from build123d import *

# Parameters (mm, degrees)
CROQUIS2_W                 = 25
CROQUIS2_H                 = 50
SALIENTE_EXTRUIR1_DEPTH    = 800
SALIENTE_EXTRUIR1_2_DEPTH  = 800
SALIENTE_EXTRUIR1_3_DEPTH  = 800
SALIENTE_EXTRUIR1_4_DEPTH  = 800
CROQUIS3_W                 = 25
CROQUIS3_H                 = 50
SALIENTE_EXTRUIR2_DEPTH    = 230
CROQUIS4_W                 = 25
CROQUIS4_H                 = 50
SALIENTE_EXTRUIR3_DEPTH    = 65
CROQUIS5_W                 = 25
CROQUIS5_H                 = 50
SALIENTE_EXTRUIR4_DEPTH    = 65
CROQUIS6_W                 = 25
CROQUIS6_H                 = 50
SALIENTE_EXTRUIR5_DEPTH    = 800
CROQUIS7_W                 = 25
CROQUIS7_H                 = 50
SALIENTE_EXTRUIR6_DEPTH    = 270
CROQUIS8_W                 = 25
CROQUIS8_H                 = 50
SALIENTE_EXTRUIR7_DEPTH    = 180
CROQUIS9_W                 = 625
CROQUIS9_H                 = 180
CROQUIS9_W_2               = 125
CORTAR_EXTRUIR1_DEPTH      = 201
CORTAR_EXTRUIR1_DEPTH_BACK = 201


with BuildPart() as part:
    # Croquis2 → Saliente-Extruir1 (new body)
    with BuildSketch(Plane.XY):
        with Locations((-187.5, 25)):
            Rectangle(CROQUIS2_W, CROQUIS2_H)
    extrude(amount=SALIENTE_EXTRUIR1_DEPTH)



with BuildPart() as body_2:
    # Croquis2 → Saliente-Extruir1 2 (new body)
    with BuildSketch(Plane.XY):
        with Locations((187.5, 25)):
            Rectangle(CROQUIS2_W, CROQUIS2_H)
    extrude(amount=SALIENTE_EXTRUIR1_2_DEPTH)


with BuildPart() as body_3:
    # Croquis2 → Saliente-Extruir1 3 (new body)
    with BuildSketch(Plane.XY):
        with Locations((-122.5, 25)):
            Rectangle(CROQUIS2_W, CROQUIS2_H)
    extrude(amount=SALIENTE_EXTRUIR1_3_DEPTH)



with BuildPart() as body_4:
    # Croquis2 → Saliente-Extruir1 4 (new body)
    with BuildSketch(Plane.XY):
        with Locations((122.5, 25)):
            Rectangle(CROQUIS2_W, CROQUIS2_H)
    extrude(amount=SALIENTE_EXTRUIR1_4_DEPTH)


with BuildPart() as body_3_1:
    add(body_3.part)

    add(body_4.part)  # Saliente-Extruir2 merges body 4
    # Croquis3 → Saliente-Extruir2 (add)
    with BuildSketch(Plane.XZ):
        with Locations((-122.5, 775)):
            Rectangle(CROQUIS3_W, CROQUIS3_H)
        with Locations((122.5, 775)):
            Rectangle(CROQUIS3_W, CROQUIS3_H)
        with Locations((-122.5, 25)):
            Rectangle(CROQUIS3_W, CROQUIS3_H)
        with Locations((122.5, 25)):
            Rectangle(CROQUIS3_W, CROQUIS3_H)
    extrude(amount=-SALIENTE_EXTRUIR2_DEPTH)


with BuildPart() as part_1:
    add(part.part)

    add(body_3_1.part)  # Saliente-Extruir3 merges body 3
    # Croquis4 → Saliente-Extruir3 (add)
    with BuildSketch(Plane.ZY.offset(200)):
        with Locations((12.5, 25)):
            Rectangle(CROQUIS4_W, CROQUIS4_H)
        with Locations((787.5, 25)):
            Rectangle(CROQUIS4_W, CROQUIS4_H)
    extrude(amount=-SALIENTE_EXTRUIR3_DEPTH)


    add(body_2.part)  # Saliente-Extruir4 merges body 2
    # Croquis5 → Saliente-Extruir4 (add)
    with BuildSketch(Plane(origin=(200, 0, 0), x_dir=(0, 0, -1), z_dir=(1, 0, 0))):
        with Locations((-787.5, 25)):
            Rectangle(CROQUIS5_W, CROQUIS5_H)
        with Locations((-12.5, 25)):
            Rectangle(CROQUIS5_W, CROQUIS5_H)
    extrude(amount=-SALIENTE_EXTRUIR4_DEPTH)

    # Croquis6 → Saliente-Extruir5 (add)
    with BuildSketch(Plane.XY.offset(800)):
        with Locations((-122.5, 205)):
            Rectangle(CROQUIS6_W, CROQUIS6_H)
        with Locations((122.5, 205)):
            Rectangle(CROQUIS6_W, CROQUIS6_H)
    extrude(amount=-SALIENTE_EXTRUIR5_DEPTH)

    # Croquis7 → Saliente-Extruir6 (add)
    with BuildSketch(Plane(origin=(135, 0, 0), x_dir=(0, 0, -1), z_dir=(1, 0, 0))):
        with Locations((-637.5, 205)):
            Rectangle(CROQUIS7_W, CROQUIS7_H)
    extrude(amount=-SALIENTE_EXTRUIR6_DEPTH)

    # Croquis8 → Saliente-Extruir7 (add)
    with BuildSketch(Plane(origin=(0, 230, 0), x_dir=(1, 0, 0), z_dir=(0, 1, 0))):
        with Locations((-122.5, -650)):
            Rectangle(CROQUIS8_W, CROQUIS8_H)
        with Locations((122.5, -650)):
            Rectangle(CROQUIS8_W, CROQUIS8_H)
    extrude(amount=-SALIENTE_EXTRUIR7_DEPTH)

    # Croquis9 → Cortar-Extruir1 (cut, two sides)
    with BuildSketch(Plane(origin=(0, 0, 0), x_dir=(0, 0, -1), z_dir=(1, 0, 0))) as cortar_extruir1_sk:
        with Locations((-312.5, 140)):
            Rectangle(CROQUIS9_W, CROQUIS9_H)
        with Locations((-737.5, 140)):
            Rectangle(CROQUIS9_W_2, CROQUIS9_H)
    extrude(amount=CORTAR_EXTRUIR1_DEPTH, mode=Mode.SUBTRACT)
    extrude(cortar_extruir1_sk.sketch, amount=-CORTAR_EXTRUIR1_DEPTH_BACK, mode=Mode.SUBTRACT)


solid = part_1.part
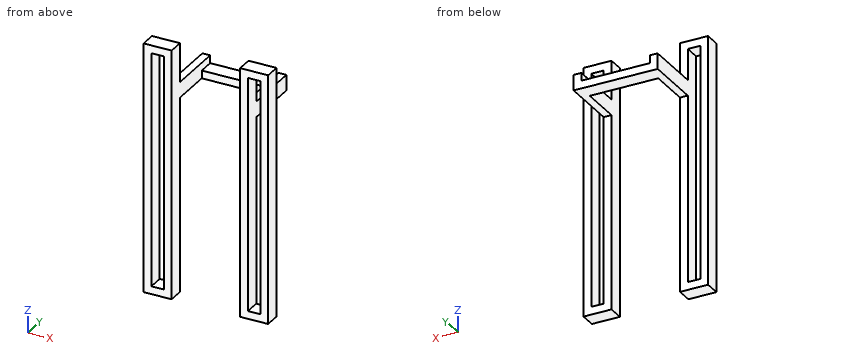
Part model, mm, in its own coordinate system. Coordinates: 2 decimals unless noted, no trailing zeros. Loops run counter-clockwise (first coordinate to the right, second up) from the corner with the lowest first, then second, coordinate; pieces in that order, holes last. Notation, with made-up numbers: (-1, -23) - (16, -23) arc R6 cw to (16, -17) - close; hole circle Ø4 at (76, 61). An arc over 180 degrees is marked (long way). Write each question's results on one line, items separated by ' | '. Start each with the question number.
Q1. Probe line 1 along X through (y, z) = (27.5, 610); line 2 along X through (y, z) = (110, 636); line 3 along Z through (x, y) = (-44.5, 188). List the from-to ranges inside material, lowest first.
Q2. Drop flat-ended pins along their axis: pin 1 Ø20 at (x, z) = (6, 633) entering from -Y; pin 2 Ø1 at (x, z) = (130.5, 586) entering from +Y; pin 3 Ø1.5 at (x, y) = (-130, 180.5) entering from +Z. Give the stop position or say it passes through.
Q3. Slice it at A-A on y = 139. Give the cut face in (x, z), and give its area (3 significant figures).
Q4. Slice it at C-C on x = 151. Give the cut face in (y, z).
Q5. Slice it at D-D on y = 216. Give the cut face in (x, z), and give its area (3 significant figures).
Q6. Slice it at B-B on z = 101. Give the cut face in (x, y), and give its area (3 significant figures).
Answer:
1) line 1: x = -200 to -175, -135 to -110, 110 to 135, 175 to 200 | line 2: x = -135 to -110, 110 to 135 | line 3: z = 625 to 650
2) pin 1: stops at y = 180 | pin 2: stops at y = 50 | pin 3: stops at z = 675
3) outline: (-135, 625) - (-110, 625) - (-110, 675) - (-135, 675) - close; (110, 625) - (135, 625) - (135, 675) - (110, 675) - close | area: 2,500 mm2
4) outline: (0, 0) - (50, 0) - (50, 25) - (0, 25) - close; (0, 775) - (50, 775) - (50, 800) - (0, 800) - close
5) outline: (-135, 625) - (135, 625) - (135, 675) - (110, 675) - (110, 650) - (-110, 650) - (-110, 675) - (-135, 675) - close | area: 8,000 mm2
6) outline: (-200, 0) - (-175, 0) - (-175, 50) - (-200, 50) - close; (-135, 0) - (-110, 0) - (-110, 50) - (-135, 50) - close; (110, 0) - (135, 0) - (135, 50) - (110, 50) - close; (175, 0) - (200, 0) - (200, 50) - (175, 50) - close | area: 5,000 mm2
